CAD build for the part. Positions are in the model's coordinates, mm. A direction names the side the tool comes from. Coordinates: 2 decimals unless noted, no trailing zeros. Order: outer loops, then holes, each group sorted by start corner. A loop starts at its lowest first (then second) coordinate and runs counter-clockwise, first axis right, second up. Notation, with made-up numbers: (-21, 62) -> (-15, 62) arc R18 cw to (-15, 73) -> close; hole circle Ø8 at (23, 34.5). An arc over 180 degrees is marked (long way). Use one line per item in the form item = value. Start each with the question number.
from build123d import *

# Parameters (mm, degrees)
SKETCH1_R           = 2.5
BOSS_EXTRUDE1_DEPTH = 482.6
SKETCH2_W           = 35.989521226
SKETCH2_H           = 397.523683421
CUT_EXTRUDE1_DEPTH  = 21


with BuildPart() as part:
    # Sketch1 → Boss-Extrude1 (new body)
    with BuildSketch(Plane.XY):
        with BuildLine():
            Line((-5.63, 10), (-9, 10))
            ThreePointArc((-9, 10), (-9.707106781, 9.707106781), (-10, 9))
            Line((-10, 9), (-10, 5.63))
            Line((-10, 5.63), (-10, 3.6))
            Line((-10, 3.6), (-8.5, 3.6))
            Line((-8.5, 3.6), (-8.5, 5.63))
            Line((-8.5, 5.63), (-6.402046573, 5.63))
            Line((-6.402046573, 5.63), (-3.95, 3.177953427))
            Line((-3.95, 3.177953427), (-3.95, -3.088580227))
            Line((-3.95, -3.088580227), (-6.491419773, -5.63))
            Line((-6.491419773, -5.63), (-8.5, -5.63))
            Line((-8.5, -5.63), (-8.5, -3.6))
            Line((-8.5, -3.6), (-10, -3.6))
            Line((-10, -3.6), (-10, -5.63))
            Line((-10, -5.63), (-10, -9))
            ThreePointArc((-10, -9), (-9.707106781, -9.707106781), (-9, -10))
            Line((-9, -10), (-5.63, -10))
            Line((-5.63, -10), (-3.6, -10))
            Line((-3.6, -10), (-3.6, -8.5))
            Line((-3.6, -8.5), (-5.63, -8.5))
            Line((-5.63, -8.5), (-5.63, -6.402046573))
            Line((-5.63, -6.402046573), (-3.177953427, -3.95))
            Line((-3.177953427, -3.95), (2.991333041, -3.95))
            Line((2.991333041, -3.95), (5.63, -6.588666959))
            Line((5.63, -6.588666959), (5.63, -8.5))
            Line((5.63, -8.5), (3.6, -8.5))
            Line((3.6, -8.5), (3.6, -10))
            Line((3.6, -10), (5.63, -10))
            Line((5.63, -10), (9, -10))
            ThreePointArc((9, -10), (9.707106781, -9.707106781), (10, -9))
            Line((10, -9), (10, -5.63))
            Line((10, -5.63), (10, -3.6))
            Line((10, -3.6), (8.5, -3.6))
            Line((8.5, -3.6), (8.5, -5.63))
            Line((8.5, -5.63), (6.491419773, -5.63))
            Line((6.491419773, -5.63), (3.95, -3.088580227))
            Line((3.95, -3.088580227), (3.95, 3.177953427))
            Line((3.95, 3.177953427), (6.402046573, 5.63))
            Line((6.402046573, 5.63), (8.5, 5.63))
            Line((8.5, 5.63), (8.5, 3.6))
            Line((8.5, 3.6), (10, 3.6))
            Line((10, 3.6), (10, 5.63))
            Line((10, 5.63), (10, 9))
            ThreePointArc((10, 9), (9.707106781, 9.707106781), (9, 10))
            Line((9, 10), (5.63, 10))
            Line((5.63, 10), (3.6, 10))
            Line((3.6, 10), (3.6, 8.5))
            Line((3.6, 8.5), (5.63, 8.5))
            Line((5.63, 8.5), (5.63, 6.588666959))
            Line((5.63, 6.588666959), (2.991333041, 3.95))
            Line((2.991333041, 3.95), (-3.177953427, 3.95))
            Line((-3.177953427, 3.95), (-5.63, 6.402046573))
            Line((-5.63, 6.402046573), (-5.63, 8.5))
            Line((-5.63, 8.5), (-3.6, 8.5))
            Line((-3.6, 8.5), (-3.6, 10))
            Line((-3.6, 10), (-5.63, 10))
        make_face()
        Circle(SKETCH1_R, mode=Mode.SUBTRACT)
    extrude(amount=BOSS_EXTRUDE1_DEPTH)

    # Sketch2 → Cut-Extrude1 (cut, through all)
    with BuildSketch(Plane(origin=(0, 10, 0), x_dir=(1, 0, 0), z_dir=(0, 1, 0))):
        with Locations((3.85907628, -300.361841711)):
            Rectangle(SKETCH2_W, SKETCH2_H)
    extrude(amount=-CUT_EXTRUDE1_DEPTH, mode=Mode.SUBTRACT)


solid = part.part
1) 3-axis set-ups, long thin cutter, end or side, ignore diameter. For faces 1 (the face through (-3.95, 0, 50)), 2 (the face through (-7, -5.63, 50)), 3 (the face through (-6, -10, 50)): which of +Z, -Z, +X, -X, +Y, -Y reach the whole face in a straight line?
2) Cut at A-A on x = 0. Give the cut face in (y, z), then the cut area to 3 significant figures.
3) Two-plate mould, pull along Y, no slides. Class faces 4 (the face through (0, 3.95, 50)), 5 (the face through (6, -10, 50)), 6 (the face through (-5, 8.5, 50)): released by +Y, released by -Y, zero draft, split by the parting line, or undercut.
4) Probe L1, parallel to Y at x = 8, z = 47.5; L2, parallel to X at y = 0.25, z = 64. List the from-to ranges inside material, lowest first.
5) Drop flat-ended pins along their axis: P1, Ø12, axis at x = -2, y = 7.5, coming from the +Z side; P2, Ø1.5, axis at y = 1, z = 85.5, coming from the +X side; P3, Ø3, axis at y = 0.5, z = 26, coming from the -X side; P4, Ø3, axis at x = 0.5, z = 47.5, coming from the +Y side. Give the stop position or say it passes through.
Values follow:
q1.face_1 = +Z, -Z, -X
q1.face_2 = +Z, -Z
q1.face_3 = +Z, -Z, +X, -X, -Y
q2.outline = (-3.95, 0) -> (-2.5, 0) -> (-2.5, 101.6) -> (-3.95, 101.6) -> close; (2.5, 0) -> (3.95, 0) -> (3.95, 101.6) -> (2.5, 101.6) -> close
q2.area = 295 mm^2
q3.face_4 = released by +Y
q3.face_5 = released by -Y
q3.face_6 = undercut
q4.L1 = -10 to -5.63, 5.63 to 10
q4.L2 = -3.95 to -2.49, 2.49 to 3.95
q5.P1 = 101.6
q5.P2 = 3.95
q5.P3 = -3.95
q5.P4 = 3.95
